from build123d import *

# Parameters (mm, degrees)
SKETCH1_W               = 17.7
SKETCH1_H               = 60
BOSS_EXTRUDE1_DEPTH     = 3
SKETCH2_W               = 3
SKETCH2_H               = 38.75
CUT_EXTRUDE1_DEPTH      = 56.240991234
CUT_EXTRUDE2_DEPTH      = 56.240991234
CUT_EXTRUDE3_DEPTH      = 2
SKETCH5_W               = 11.7
SKETCH5_H               = 10
BOSS_EXTRUDE2_DEPTH     = 2
CUT_EXTRUDE4_DEPTH      = 56.385621893
CUT_EXTRUDE4_DEPTH_BACK = 56.385621893
SKETCH6_R               = 2.35
FILLET1_R               = 2
FILLET2_R               = 2
FILLET3_R               = 2
FILLET4_R               = 2


with BuildPart() as part:
    # Sketch1 → Boss-Extrude1 (new body)
    with BuildSketch(Plane.XY):
        with Locations((-34.564285714, 4.025974026)):
            Rectangle(SKETCH1_W, SKETCH1_H)
    extrude(amount=BOSS_EXTRUDE1_DEPTH)

    # Sketch2 → Cut-Extrude1 (cut, through all)
    with BuildSketch(Plane.XY.offset(3)):
        with Locations((-41.914285714, -6.599025974)):
            Rectangle(SKETCH2_W, SKETCH2_H)
        with Locations((-27.214285714, -6.599025974)):
            Rectangle(SKETCH2_W, SKETCH2_H)
    extrude(amount=-CUT_EXTRUDE1_DEPTH, mode=Mode.SUBTRACT)

    # Sketch3 → Cut-Extrude2 (cut, through all)
    with BuildSketch(Plane.XY.offset(3)):
        with BuildLine():
            Line((-28.714285714, 25.525974026), (-38.714285714, 25.525974026))
            ThreePointArc((-38.714285714, 25.525974026), (-39.964285714, 26.775974026), (-38.714285714, 28.025974026))
            Line((-38.714285714, 28.025974026), (-28.714285714, 28.025974026))
            ThreePointArc((-28.714285714, 28.025974026), (-27.464285714, 26.775974026), (-28.714285714, 25.525974026))
        make_face()
    extrude(amount=-CUT_EXTRUDE2_DEPTH, mode=Mode.SUBTRACT)

    # Sketch4 → Cut-Extrude3 (cut)
    with BuildSketch(Plane.XY.offset(3)):
        with BuildLine():
            Line((-38.714285714, 28.775974026), (-28.714285714, 28.775974026))
            ThreePointArc((-28.714285714, 28.775974026), (-26.714285714, 26.775974026), (-28.714285714, 24.775974026))
            Line((-28.714285714, 24.775974026), (-38.714285714, 24.775974026))
            ThreePointArc((-38.714285714, 24.775974026), (-40.714285714, 26.775974026), (-38.714285714, 28.775974026))
        make_face()
    extrude(amount=-CUT_EXTRUDE3_DEPTH, mode=Mode.SUBTRACT)

    # Sketch5 → Boss-Extrude2 (add)
    with BuildSketch(Plane(origin=(0, 0, 0), x_dir=(-1, 0, 0), z_dir=(0, 0, -1))):
        with Locations((34.564285714, -20.974025974)):
            Rectangle(SKETCH5_W, SKETCH5_H)
    extrude(amount=BOSS_EXTRUDE2_DEPTH)

    # Sketch6 → Cut-Extrude4 (cut, two sides: drawn at the far end of the back side and taken through both)
    with BuildSketch(Plane(origin=(0, 0, -2), x_dir=(-1, 0, 0), z_dir=(0, 0, -1)).offset(-CUT_EXTRUDE4_DEPTH_BACK)):
        with Locations((34.564285714, -20.974025974)):
            Circle(SKETCH6_R)
    extrude(amount=CUT_EXTRUDE4_DEPTH + CUT_EXTRUDE4_DEPTH_BACK, mode=Mode.SUBTRACT)

    # Fillet1
    fillet1_edges = [part.edges().sort_by_distance(p)[0] for p in [
        (-34.564285714, -25.974025974, -2),
    ]]
    fillet(fillet1_edges, radius=FILLET1_R)

    # Fillet2
    fillet2_edges = [part.edges().sort_by_distance(p)[0] for p in [
        (-34.564285714, -15.974025974, -2),
    ]]
    fillet(fillet2_edges, radius=FILLET2_R - 0.0001)  # a hair under: the kernel refuses the full size

    # Fillet3
    fillet3_edges = [part.edges().sort_by_distance(p)[0] for p in [
        (-28.714285714, -25.974025974, 1.5),
        (-28.714285714, -25.388239536, -1.414213562),
        (-28.714285714, -20.973975974, -2),
        (-28.714285714, -16.559783122, -1.414242852),
    ]]
    fillet(fillet3_edges, radius=FILLET3_R - 0.0001)  # a hair under: the kernel refuses the full size

    # Fillet4
    fillet4_edges = [part.edges().sort_by_distance(p)[0] for p in [
        (-40.414285714, -20.973975974, -2),
        (-40.414285714, -25.974025974, 1.5),
        (-40.414285714, -25.388239536, -1.414213562),
        (-40.414285714, -16.559783122, -1.414242852),
    ]]
    fillet(fillet4_edges, radius=FILLET4_R - 0.0001)  # a hair under: the kernel refuses the full size


solid = part.part
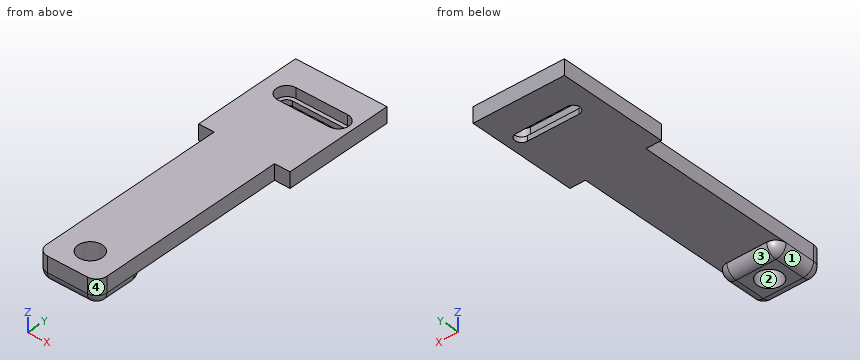
Source: CAD feature listing. Evaluate the final solid. Frame: model axes, mm. Face numbers are marked on the shaded views. Give positions to 0.01 mm unless a question says otherwise; leave off trailing zeros. Write each loop counter-clockwise with the first axis right and the second up, starting at its lowest first coordinate (ties: lowest second). Pieces come first, ordered by that corner, then holes. Notation, with made-up numbers: (4.25, 22) - (15.25, 22) arc R12 cw to (15.25, 29) - close; hole circle Ø3 at (-18.5, -29.5). An arc over 180 degrees is marked (long way). Write item = value, one per line. Start each with the question number.
Q1. Cut plane C-C, the plane x = -34.5. Give the number of separate pieces and of enclosed holes in the cut face, then the cut area to 3 significant figures.
Q2. Pin query (flat end, axial travel): pin 1 Ø1 at (y, z) = (-16.5, 2) entering from +X; pin 2 Ø5.5 at (x, y) = (-37.5, 11) entering from -Z; pin 3 Ø2.5 at (x, z) = (-42, 2) entering from -Y. Return the tip coordinate at first contact, or that it passes through.
Q3. Draft query along X for the marked faces 1, 2, 3 and 4. Return one class per face: +X half, -X half, draft (parallel to the pull), parting line (faces both ways), or undercut.
Q4. Cut plane A-A, the plane y = -20. Return loops of the section in (x, z), then the cut area to 3 significant figures.
Q5. Cut plane D-D, the plane z = 1.55. Return loops of the section in (x, y), then the cut area to 3 significant figures.
Q6. Material intervals for probe 1 along Y at (x, z) = (-37.25, 0.2); probe 2 along Y at (x, z) = (-36, 2.35); probe 3 along Y at (x, z) = (-33, 1.7), sorted ascending.
Computed values:
q1.separate_pieces = 3
q1.enclosed_holes = 0
q1.area = 164 mm²
q2.pin_1 = -28.71
q2.pin_2 = 0
q2.pin_3 = 12.78
q3.face_1 = -X half
q3.face_2 = undercut
q3.face_3 = draft
q3.face_4 = +X half
q4.outline = (-40.41, 0) arc R2 ccw to (-38.41, -2) - (-36.7, -2) - (-36.7, 3) - (-40.41, 3) - close; (-32.43, -2) - (-30.71, -2) arc R2 ccw to (-28.71, 0) - (-28.71, 3) - (-32.43, 3) - close
q4.area = 35.4 mm²
q5.outline = (-43.41, 12.78) - (-40.41, 12.78) - (-40.41, -23.97) arc R2 ccw to (-38.41, -25.97) - (-30.71, -25.97) arc R2 ccw to (-28.71, -23.97) - (-28.71, 12.78) - (-25.71, 12.78) - (-25.71, 34.03) - (-43.41, 34.03) - close; hole (-38.71, 24.78) - (-28.71, 24.78) arc R2 ccw to (-28.71, 28.78) - (-38.71, 28.78) arc R2 ccw to start; hole circle Ø4.7 at (-34.56, -20.97)
q5.area = 758 mm²
q6.probe_1 = -25.97 to 25.53, 28.03 to 34.03
q6.probe_2 = -25.97 to -22.83, -19.11 to 24.78, 28.78 to 34.03
q6.probe_3 = -25.97 to -22.73, -19.22 to 24.78, 28.78 to 34.03
